Input: part model. Units: mm. Frame: model coordinates. Round coordinates to 2 decimals unless told otherwise and drop trailing zeros. Loops run counter-clockwise (first coordinate to the right, second up) from the corner with the lowest first, then second, coordinate; pieces in that order, holes last. Notation, with made-up numbers: M 75.25,-9.75 L 105.25,-9.75 A22 ccw 105.25,9.25 Z; hole C -18.75,21.5 d11. An arc over 180 degrees is marked long. Put each result on its own line as item: value. Start each with the question number.
1) Section B-B on z = -4.5. State how many separate pieces and enclosed holes the cut face has, plus the area to 3 significant figures.
2) Pin query (flat end, axial travel): pin 1 (5 mm diameter, centred on x = -8.06, y = -37.72, fed in from +Z); pin 2 (2 mm diameter, centred on x = 20.5, z = -3, fed in from -Y). Return the tip coordinate at first contact, or that it passes through.
3) Line query: probe 1 along X at (y, z) = (34, -1.25); probe 2 along X at (y, z) = (-36, -3.25); probe 3 along Y at (x, z) = (25, -3.5). Output: solid intervals per line, ascending.
4) Section A-A on x = 6. Output: boundary loops of the cut face in (y, z), plus the area to 3 significant figures.
5) Section C-C on y = -13. Output: boundary loops of the cut face in (x, z), plus the area to 3 significant figures.
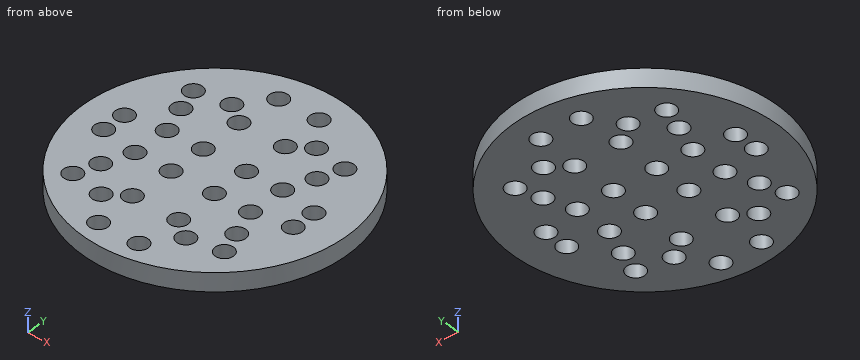
from build123d import *

# Parameters (mm, degrees)
F0_R     = 45.543939
F2_DEPTH = 6.35
F3_D     = 6.35


with BuildPart() as f2:
    # F0 (on Top) → F2 (new body)
    with BuildSketch(Plane.XY):
        Circle(F0_R)
    extrude(amount=-F2_DEPTH)

    # F3 (through all)
    with Locations(Plane.XY):
        with Locations((-9.101805, -22.868802), (-15.81638, -27.738158), (-27.532594, -25.683472), (-24.809956, -17.553446), (-8.565614, -7.831892), (-21.215289, -7.831892), (13.849741, -27.738158), (25.565955, -25.683472), (22.843317, -17.553446), (7.135166, -22.868802), (6.096926, -37.724978), (-8.063565, -37.724978), (6.598975, -7.831892), (19.24865, -7.831892), (32.221985, -5.533049), (32.221985, 2.85738), (19.24865, 5.156223), (6.598975, 5.156223), (7.135166, 20.193133), (13.849741, 25.062489), (25.565955, 23.007803), (22.843317, 14.877777), (6.096926, 35.049309), (-8.565614, 5.156223), (-21.215289, 5.156223), (-34.188624, 2.85738), (-34.188624, -5.533049), (-9.101805, 20.193133), (-24.809956, 14.877777), (-15.81638, 25.062489), (-27.532594, 23.007803), (-8.063565, 35.049309)):
            Hole(F3_D / 2)


solid = f2.part
Geometry results:
1. separate pieces: 1
1. enclosed holes: 32
1. area: 5,500 mm²
2. pin 1: passes through
2. pin 2: stops at y = -41.16
3. probe 1: x = -30.3 to -11.06, -5.07 to 3.1, 9.09 to 30.3
3. probe 2: x = -27.9 to -10.73, -5.4 to 3.43, 8.76 to 27.9
3. probe 3: y = -38.07 to -28.81, -22.56 to -19.88, -15.22 to 12.55, 17.21 to 19.88, 26.13 to 38.07
4. outline: M -45.15,-6.35 L -40.9,-6.35 L -40.9,0 L -45.15,0 Z; M -34.55,-6.35 L -25.83,-6.35 L -25.83,0 L -34.55,0 Z; M -19.9,-6.35 L -10.95,-6.35 L -10.95,0 L -19.9,0 Z; M -4.71,-6.35 L 2.04,-6.35 L 2.04,0 L -4.71,0 Z; M 8.27,-6.35 L 17.23,-6.35 L 17.23,0 L 8.27,0 Z; M 23.16,-6.35 L 31.88,-6.35 L 31.88,0 L 23.16,0 Z; M 38.22,-6.35 L 45.15,-6.35 L 45.15,0 L 38.22,0 Z
4. area: 338 mm²
5. outline: M -43.65,-6.35 L 43.65,-6.35 L 43.65,0 L -43.65,0 Z
5. area: 554 mm²
